Input: part model. Units: mm. Frame: model coordinates. A direction names the side the tool comes from. Round coordinates to 2 decimals unless told otherwise and drop trailing zeros. Order: outer loops, then holes, each group sorted by start corner. A loop starts at its lowest first (then second) coordinate and runs counter-clockwise, first axis right, second up. Notation, with made-up numbers: (86.25, 46.25) -> (144.25, 46.25) arc R11 cw to (144.25, 52.25) -> close; hole circle Ø7 at (-19.5, 48.25). An arc over 180 degrees is marked (long way). Answer as CSV lines item,"result". Start each with the question number.
1) Line query: L1, parallel to Y at x = 29.5, z = 8; L2, parallel to X at y = 22, z = 4.5. Output: solid intervals per line, ascending.
2) Section query C-C, the plane y = 33.5. Output: boundary loops of the cut face in (x, z), and give its area (3 significant figures).
3) Mould query, pull axis Y, two halves, no side actions, for faces 3 (the face through (100, 37, 5)), 4 (the face through (49, 0, 5)), 5 (the face through (51, 75, 5)), 6 (the face through (30, 55, 5)). Classes: +Y half, -Y half, draft (parallel to the pull), parting line (faces both ways), or undercut.
4) Access query for faces 1 (the face through (60, 37, 5)), 2 (the face through (0, 10, 5)). Directions: +Z, -Z, +X, -X, +Y, -Y. A direction counts if a zero-diameter tool reaches every point of the face in a straight line with its end or side. Return the directions, or none.
5) Section query B-B, the plane z = 1.25. Output: boundary loops of the cut face in (x, y), and give its area (3 significant figures).
6) Section query A-A, the plane x = 48.5. Output: boundary loops of the cut face in (y, z), and give its area (3 significant figures).
7) First-contact query: P1, Ø5, axis at y = 52, z = 4.5, coming from the -X side. Flat tip, straight axial feed; report the tip coordinate or a pass-through.
```python
from build123d import *

# Parameters (mm, degrees)
F0_W     = 40
F0_H     = 35
F1_DEPTH = 10
F3_DEPTH = 10


with BuildPart() as f1:
    # F0 (on Top) → F1 (new body)
    with BuildSketch(Plane.XY):
        Polygon((0, 75), (0, 55), (60, 55), (100, 55), (100, 75), align=None)
        with Locations((80, 37.5)):
            Rectangle(F0_W, F0_H)
        Polygon((0, 20), (0, 0), (100, 0), (100, 20), (60, 20), align=None)
    extrude(amount=F1_DEPTH)

    # F2 (on face) → F3 (join, through all)
    with BuildSketch(Plane.XY.offset(10)):
        with BuildLine():
            ThreePointArc((0, 68), (6.9741670742, 72.626784841), (15, 75))
            Line((15, 75), (0, 75))
            Line((0, 75), (0, 68))
        make_face()
        with BuildLine():
            ThreePointArc((15, 0), (6.7778411295, 1.9525167061), (0, 7))
            Line((0, 7), (0, 0))
            Line((0, 0), (15, 0))
        make_face()
    extrude(amount=-F3_DEPTH)


solid = f1.part
```
Findings:
1,L1,"y = 0 to 20, 55 to 75"
1,L2,"x = 60 to 100"
2,outline,"(60, 0) -> (100, 0) -> (100, 10) -> (60, 10) -> close"
2,area,"400 mm^2"
3,face 3,"draft"
3,face 4,"-Y half"
3,face 5,"+Y half"
3,face 6,"undercut"
4,face 1,"+Z, -Z, -X"
4,face 2,"+Z, -Z, -X, +Y, -Y"
5,outline,"(0, 0) -> (100, 0) -> (100, 75) -> (0, 75) -> (0, 55) -> (60, 55) -> (60, 20) -> (0, 20) -> close"
5,area,"5,400 mm^2"
6,outline,"(0, 0) -> (20, 0) -> (20, 10) -> (0, 10) -> close; (55, 0) -> (75, 0) -> (75, 10) -> (55, 10) -> close"
6,area,"400 mm^2"
7,P1,"stops at x = 60"
